```python
from build123d import *

# Parameters (mm, degrees)
F1_DEPTH = 50


with BuildPart() as f1:
    # F0 (on Top) → F1 (new body)
    with BuildSketch(Plane.XY):
        Polygon((-567.647423, -242.966514), (-567.647423, -272.966514), (-465.647423, -272.966514), (-465.647423, -242.966514), (-467.647423, -242.966514), (-467.647423, -262.966514), (-469.647423, -262.966514), (-469.647423, -242.966514), (-471.647423, -242.966514), (-471.647423, -262.966514), (-473.647423, -262.966514), (-473.647423, -242.966514), (-475.647423, -242.966514), (-475.647423, -262.966514), (-477.647423, -262.966514), (-477.647423, -242.966514), (-479.647423, -242.966514), (-479.647423, -262.966514), (-481.647423, -262.966514), (-481.647423, -242.966514), (-483.647423, -242.966514), (-483.647423, -262.966514), (-485.647423, -262.966514), (-485.647423, -242.966514), (-487.647423, -242.966514), (-487.647423, -262.966514), (-489.647423, -262.966514), (-489.647423, -242.966514), (-491.647423, -242.966514), (-491.647423, -262.966514), (-493.647423, -262.966514), (-493.647423, -242.966514), (-495.647423, -242.966514), (-495.647423, -262.966514), (-497.647423, -262.966514), (-497.647423, -242.966514), (-499.647423, -242.966514), (-499.647423, -262.966514), (-501.647423, -262.966514), (-501.647423, -242.966514), (-503.647423, -242.966514), (-503.647423, -262.966514), (-505.647423, -262.966514), (-505.647423, -242.966514), (-507.647423, -242.966514), (-507.647423, -262.966514), (-509.647423, -262.966514), (-509.647423, -242.966514), (-511.647423, -242.966514), (-511.647423, -262.966514), (-513.647423, -262.966514), (-513.647423, -242.966514), (-515.647423, -242.966514), (-515.647423, -262.966514), (-517.647423, -262.966514), (-517.647423, -242.966514), (-519.647423, -242.966514), (-519.647423, -262.966514), (-521.647423, -262.966514), (-521.647423, -242.966514), (-523.647423, -242.966514), (-523.647423, -262.966514), (-525.647423, -262.966514), (-525.647423, -242.966514), (-527.647423, -242.966514), (-527.647423, -262.966514), (-529.647423, -262.966514), (-529.647423, -242.966514), (-531.647423, -242.966514), (-531.647423, -262.966514), (-533.647423, -262.966514), (-533.647423, -242.966514), (-535.647423, -242.966514), (-535.647423, -262.966514), (-537.647423, -262.966514), (-537.647423, -242.966514), (-539.647423, -242.966514), (-539.647423, -262.966514), (-541.647423, -262.966514), (-541.647423, -242.966514), (-543.647423, -242.966514), (-543.647423, -262.966514), (-545.647423, -262.966514), (-545.647423, -242.966514), (-547.647423, -242.966514), (-547.647423, -262.966514), (-549.647423, -262.966514), (-549.647423, -242.966514), (-551.647423, -242.966514), (-551.647423, -262.966514), (-553.647423, -262.966514), (-553.647423, -242.966514), (-555.647423, -242.966514), (-555.647423, -262.966514), (-557.647423, -262.966514), (-557.647423, -242.966514), (-559.647423, -242.966514), (-559.647423, -262.966514), (-561.647423, -262.966514), (-561.647423, -242.966514), (-563.647423, -242.966514), (-563.647423, -262.966514), (-565.647423, -262.966514), (-565.647423, -242.966514), align=None)
    extrude(amount=F1_DEPTH)


solid = f1.part
```
Work out the finished part from the listing and answer in its coordinate system (mm). A direction names the side the tool comes from. Coordinates: 2 decimals unless noted, no trailing zeros. Use a Markdown table: item, result.
Item 1: Find section A-A, the plane y = -247. State how many separate pieces and enclosed holes the cut face has, and give its area (3 significant figures).
Evaluation:
| item | result |
|---|---|
| separate pieces | 26 |
| enclosed holes | 0 |
| area | 2,600 mm2 |
Item 2: Given pin 1 Ø0.6 at (x, z) = (-492, 31) entering from +Y, flat-ended and moving along its own axis, determine where the tip first touches the part or whether it passes through.
Evaluation:
| item | result |
|---|---|
| pin 1 | stops at y = -262.97 |
Item 3: Consider probe 1 along Y at (x, z) = (-524, 13). Determine where the line is inside the solid, lowest interval first. Write a range as from..to.
Evaluation:
| item | result |
|---|---|
| probe 1 | y = -272.97..-262.97 |
Item 4: The mould has two halves that part along X. Classify faces 3 (the flat face through (-561.647, -253, 25)), 4 (the flat face through (-515, -242.967, 25)): +X half, -X half, draft (parallel to the pull), parting line (faces both ways), or undercut.
Evaluation:
| item | result |
|---|---|
| face 3 | undercut |
| face 4 | draft |
Item 5: For faces 1 (the flat face through (-545.647, -253, 25)), 2 (the flat face through (-517, -264, 50)), determine the directions among +Z, -Z, +X, -X, +Y, -Y from which every point of the face is accessible in a straight line to the end or side of a thin tool.
Evaluation:
| item | result |
|---|---|
| face 1 | +Z, -Z, +Y |
| face 2 | +Z, +X, -X, +Y, -Y |
